Here's how the part is built. I have some questions about the finished solid (model axes, mm). Face numbers are marked on the shaded views. A direction names the side the tool comes from. Coordinates: 2 decimals unless noted, no trailing zeros. Write each loop counter-clockwise with the first axis right and the second up, starting at its lowest first coordinate (ties: lowest second). Pieces come first, ordered by that corner, then holes. Notation, with made-up numbers: M -16.5,-36 L 11.5,-36 A29 ccw 11.5,-10 Z; hole C 86.5,-5 d9. An arc over 180 degrees is marked long. Write each question's results on one line, items separated by ' | '. Start each with the question number.
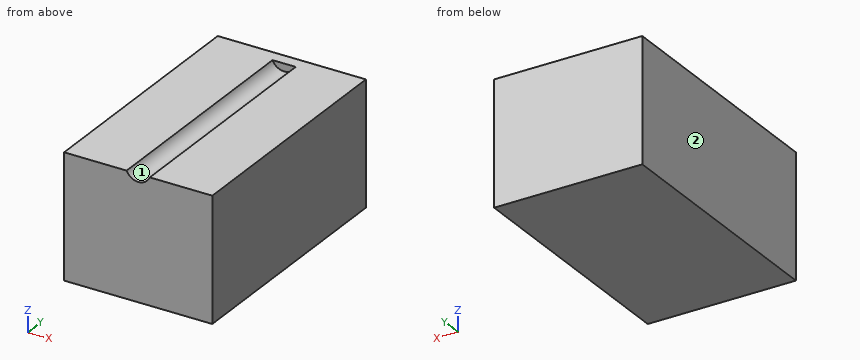
from build123d import *

# Parameters (mm, degrees)
SKETCH1_W           = 30
SKETCH1_H           = 25
BOSS_EXTRUDE1_DEPTH = 50
CUT_EXTRUDE2_START  = 2.5
SKETCH1_5_W         = 25
SKETCH1_5_H         = 20
CUT_EXTRUDE2_DEPTH  = 45
BOSS_EXTRUDE3_START = 25
SKETCH1_6_W         = 25
SKETCH1_6_H         = 20
BOSS_EXTRUDE3_DEPTH = 1
SKETCH2_R           = 2.55
CUT_EXTRUDE3_DEPTH  = 47.5
SKETCH4_W           = 25
SKETCH4_H           = 5
CUT_EXTRUDE4_DEPTH  = 1


with BuildPart() as part:
    # Sketch1 → Boss-Extrude1 (new body)
    with BuildSketch(Plane(origin=(0, 0, 0), x_dir=(1, 0, 0), z_dir=(0, 1, 0))):
        Rectangle(SKETCH1_W, SKETCH1_H)
    extrude(amount=BOSS_EXTRUDE1_DEPTH)

    # Sketch1<5> → Cut-Extrude2 (cut)
    with BuildSketch(Plane(origin=(0, 0, 0), x_dir=(1, 0, 0), z_dir=(0, 1, 0)).offset(CUT_EXTRUDE2_START)):
        Rectangle(SKETCH1_5_W, SKETCH1_5_H)
    extrude(amount=CUT_EXTRUDE2_DEPTH, mode=Mode.SUBTRACT)

    # Sketch1<6> → Boss-Extrude3 (add)
    with BuildSketch(Plane(origin=(0, 0, 0), x_dir=(1, 0, 0), z_dir=(0, 1, 0)).offset(BOSS_EXTRUDE3_START)):
        Rectangle(SKETCH1_6_W, SKETCH1_6_H)
    extrude(amount=BOSS_EXTRUDE3_DEPTH)

    # Sketch2 → Cut-Extrude3 (cut)
    with BuildSketch(Plane(origin=(0, 47.5, 0), x_dir=(-1, 0, 0), z_dir=(0, -1, 0))):
        with Locations((0, -13.5)):
            Circle(SKETCH2_R)
    extrude(amount=CUT_EXTRUDE3_DEPTH, mode=Mode.SUBTRACT)

    # Sketch4 → Cut-Extrude4 (cut)
    with BuildSketch(Plane(origin=(0, 26, 0), x_dir=(1, 0, 0), z_dir=(0, 1, 0))):
        with Locations((0, -7.5)):
            Rectangle(SKETCH4_W, SKETCH4_H)
    extrude(amount=-CUT_EXTRUDE4_DEPTH, mode=Mode.SUBTRACT)


solid = part.part
1) For the marked faces 1 and 2, which set-ups out of +Z, -Z, +X, -X, +Y, -Y let a thin tool reach every point of the face, with its end or its side?
2) I want a section at B-B, the plane y = 13. Write out the boundary of the cut face in (x, z), then the cut area to 3 significant figures.
3) For pin 1 Ø0.5 at (x, y) = (1.5, 25.5) entering from +Z, with a flat end and sliding along its axis, tell me the tip position at first contact or that it passes through.
4) I want a section at D-D, the plane z = 3.5. Write out the boundary of the cut face in (x, y), then the cut area to 3 significant figures.
5) I want a section at C-C, the plane z = 8.25. Write out the boundary of the cut face in (x, y), then the cut area to 3 significant figures.
6) I want a section at A-A, the plane x = 5.25. Write out the boundary of the cut face in (y, z).
7) Please list where these lines run through material, in increasing order: line 1 (Y direction, x = 2, z = 3.25); line 2 (X direction, y = 28, z = -9.75); line 3 (Z direction, x = -5, y = 9). Write a range as [from, to].
Output:
1) face 1: +Z, -Y | face 2: +Z, -Z, -X, +Y, -Y
2) outline: M -15,-12.5 L 15,-12.5 L 15,12.5 L 2.35,12.5 A2.55 cw -2.35,12.5 L -15,12.5 Z; hole M -12.5,-10 L 12.5,-10 L 12.5,10 L -12.5,10 Z | area: 245 mm2
3) pin 1: stops at z = 11.65
4) outline: M -15,0 L 15,0 L 15,50 L -15,50 Z; hole M -12.5,2.5 L 12.5,2.5 L 12.5,25 L -12.5,25 Z; hole M -12.5,26 L 12.5,26 L 12.5,47.5 L -12.5,47.5 Z | area: 400 mm2
5) outline: M -15,0 L 15,0 L 15,50 L -15,50 Z; hole M -12.5,2.5 L 12.5,2.5 L 12.5,47.5 L -12.5,47.5 Z | area: 375 mm2
6) outline: M 0,-12.5 L 50,-12.5 L 50,12.5 L 0,12.5 Z; hole M 2.5,-10 L 25,-10 L 25,5 L 26,5 L 26,-10 L 47.5,-10 L 47.5,10 L 2.5,10 Z
7) line 1: y = [0, 2.5], [25, 26], [47.5, 50] | line 2: x = [-15, -12.5], [12.5, 15] | line 3: z = [-12.5, -10], [10, 12.5]
